Geometry check sheet. Reference: the model listing, model coordinates, mm. Round coordinates to 2 decimals unless told otherwise and drop trailing zeros. Order: outer loops, then holes, each group sorted by start corner. A loop starts at its lowest first (then second) coordinate and runs counter-clockwise, first axis right, second up. Notation, with made-up numbers: (74, 84) - (117, 84) arc R30 cw to (117, 123) - close; hole circle Ø8 at (50.25, -6.75). An arc over 180 degrees is marked (long way). Return JSON: item names as keys, results as strings. Group by question number.
Q1. Sectioned sample at B-B, the plane z = -13. Record the cut outline in (x, y), then the cut area to 3 significant figures.
Q2. Material ranges on line 1 along X through (y, z) = (3, -12.5); line 2 along X through (y, z) = (8.5, -54); line 3 along Z through (x, y) = (-31, 0.75), recorded low to high.
Q3. Draft check along X on faces 1 (the flat face through (0, 5, -31)), 2 (the cylindrical face through (-59.273, 5.07, -12.599)), 3 (the flat face through (-20, 5, -61)), 4 (the cylindrical face through (-41.273, 5.07, -12.599)). Enter one of: pulls with the +X half, pulls with the -X half, needs draft (parallel to the pull), parting line crosses it, or undercut.
Q4. Sectioned sample at C-C, the plane y = 7.5. Give the number of separate pieces and of enclosed holes in the cut face, then the cut area to 3 significant figures.
Q5. Gauge pin test, flat end, axial feed: pin 1 Ø5 at (x, z) = (-44, -12.24) entering from -Y. Record the tip position at first contact, or that the pin passes through.
Q6. Sectioned sample at D-D, the plane x = -44. Record the cut outline in (y, z), then the cut area to 3 significant figures.
Q7. Sectioned sample at A-A, the plane x = -8. Record the cut outline in (y, z).
```python
from build123d import *

# Parameters (mm, degrees)
BOSS_EXTRUDE2_DEPTH = 10
FILLET4_R           = 40
FILLET5_R           = 2
FILLET6_R           = 2
FILLET7_R           = 2
SKETCH2_R           = 2.75
CUT_EXTRUDE1_DEPTH  = 94.386294498


with BuildPart() as part:
    # Sketch1 → Boss-Extrude2 (new body)
    with BuildSketch(Plane(origin=(0, 0, 0), x_dir=(1, 0, 0), z_dir=(0, 1, 0))):
        Polygon((-39, 61), (0, 61), (0, 0), (-70, 0), (-70, 20), (-39, 20), align=None)
    extrude(amount=BOSS_EXTRUDE2_DEPTH)

    # Fillet4
    # the kernel refuses this fillet: 40 mm, written as the material it adds along each edge
    with BuildSketch(Plane(origin=(-39, 0, -20), x_dir=(-1, 0, 0), z_dir=(0, 1, 0))) as fillet4_piece_1:
        with BuildLine():
            CenterArc((40, -38.97435054), FILLET4_R, 103.002878163, 76.997121837)
            Line((0, -38.97435054), (-0.8, -38.97435054))
            Line((-0.8, -38.97435054), (-0.8, 0))
            Line((-0.8, 0), (0, 0.8))
            ThreePointArc((0, 0.8), (15.5, 0.8), (30.82, 0.779487011))
            Line((30.82, 0.779487011), (31, 0))
        make_face()
    extrude(amount=10)

    # Fillet5
    fillet5_edges = [part.edges().sort_by_distance(p)[0] for p in [
        (0, 5, -61),
        (0, 5, 0),
        (-70, 5, 0),
    ]]
    fillet(fillet5_edges, radius=FILLET5_R)

    # Fillet6
    fillet6_edges = [part.edges().sort_by_distance(p)[0] for p in [
        (-39, 5, -61),
    ]]
    fillet(fillet6_edges, radius=FILLET6_R)

    # Fillet7
    fillet7_edges = [part.edges().sort_by_distance(p)[0] for p in [
        (-70, 5, -20),
    ]]
    fillet(fillet7_edges, radius=FILLET7_R)

    # Sketch2 → Cut-Extrude1 (cut, through all)
    with BuildSketch(Plane(origin=(0, 10, 0), x_dir=(1, 0, 0), z_dir=(0, 1, 0))):
        with Locations(Location((-9.837865554, 53.798881229, 0), (0, 0, 270))):
            Circle(SKETCH2_R)
        with Locations(Location((-31.15958497, 53.798881229, 0), (0, 0, 270))):
            Circle(SKETCH2_R)
        with Locations(Location((-31.15958497, 36.567952328, 0), (0, 0, 270))):
            Circle(SKETCH2_R)
        with Locations(Location((-9.837865554, 36.567952328, 0), (0, 0, 270))):
            Circle(SKETCH2_R)
        with Locations(Location((-8, 12.241109826, 0), (0, 0, 270))):
            Circle(SKETCH2_R)
        with Locations(Location((-26, 12.241109826, 0), (0, 0, 270))):
            Circle(SKETCH2_R)
        with Locations(Location((-44, 12.241109826, 0), (0, 0, 270))):
            Circle(SKETCH2_R)
        with Locations(Location((-62, 12.241109826, 0), (0, 0, 270))):
            Circle(SKETCH2_R)
    extrude(amount=-CUT_EXTRUDE1_DEPTH, mode=Mode.SUBTRACT)


solid = part.part
```
Reply:
{
 "1": {"outline": "(-70, 0) - (-64.64, 0) - (-64.64, 10) - (-70, 10) - close; (-59.36, 0) - (-46.64, 0) - (-46.64, 10) - (-59.36, 10) - close; (-41.36, 0) - (-28.64, 0) - (-28.64, 10) - (-41.36, 10) - close; (-23.36, 0) - (-10.64, 0) - (-10.64, 10) - (-23.36, 10) - close; (-5.36, 0) - (0, 0) - (0, 10) - (-5.36, 10) - close", "area": "489 mm^2"},
 "2": {"line 1": "-70 to -64.74, -59.26 to -46.74, -41.26 to -28.74, -23.26 to -10.74, -5.26 to 0", "line 2": "-39.31 to -33.9, -28.42 to -12.58, -7.1 to 0", "line 3": "-61 to -56.54, -51.05 to -39.31, -33.82 to 0"},
 "3": {"face 1": "pulls with the +X half", "face 2": "undercut", "face 3": "needs draft", "face 4": "undercut"},
 "4": {"separate pieces": "1", "enclosed holes": "8", "area": "3,110 mm^2"},
 "5": {"pin 1": "through"},
 "6": {"outline": "(0, -39.61) - (10, -39.61) - (10, -14.99) - (0, -14.99) - close; (0, -9.49) - (10, -9.49) - (10, 0) - (0, 0) - close", "area": "341 mm^2"},
 "7": {"outline": "(0, -61) - (10, -61) - (10, -55.84) - (0, -55.84) - close; (0, -51.75) - (10, -51.75) - (10, -38.61) - (0, -38.61) - close; (0, -34.52) - (10, -34.52) - (10, -14.99) - (0, -14.99) - close; (0, -9.49) - (10, -9.49) - (10, 0) - (0, 0) - close"}
}
